Could you check a few things on this drawing? It's one solid part, dimensions in mm from its lowest x, y, z. Coordinates: 2 decimals unless noted, no trailing zeros. Loops run counter-clockwise (first coordinate to the right, second up) from the corner with the lowest first, then second, coordinate; pieces in that order, holes last.
1) Will these pins go through, and if not, where does the flat tip stop? P1, Ø1.2, axis at x = 28.09, z = 19.61, coming from the +Y side; P2, Ø3, axis at x = 29.5, z = 16.5, coming from the +Y side.
2) Imagine slicing it at D-D on x = 29.5. Please give me the cut outline in (y, z).
3) Imagine slicing it at B-B on x = 16.5. Please give me the cut outline in (y, z).
4) Imagine slicing it at A-A on z = 16.5. Please give me the cut outline in (x, y).
5) Imagine slicing it at C-C on z = 3.5. Please give me the cut outline in (x, y).
6) If I drill on line 1 along Z through (x, y) = (29, 0.55) (1 decimal); line 2 along Z through (x, y) = (16, 0.3) (1 decimal); line 3 along X through (y, z) = (0.7, 30.5), over which ranges is the centre line in solid material (lowest first)?
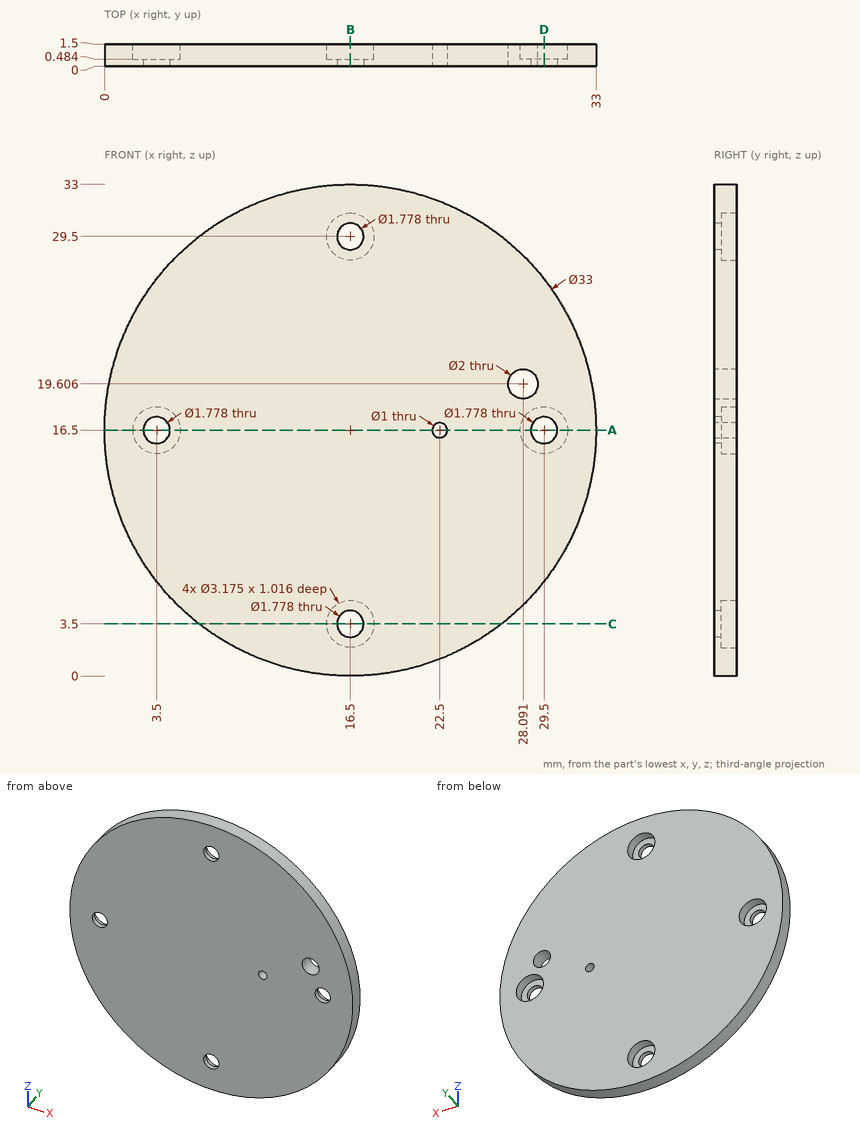
Filled in:
1. P1: passes through
1. P2: stops at y = 0.48
2. outline: (0, 6.34) - (1.5, 6.34) - (1.5, 14.91) - (0.48, 14.91) - (0.48, 15.61) - (0, 15.61) - close; (0, 17.39) - (0.48, 17.39) - (0.48, 18.09) - (1.5, 18.09) - (1.5, 26.66) - (0, 26.66) - close
3. outline: (0, 0) - (1.5, 0) - (1.5, 1.91) - (0.48, 1.91) - (0.48, 2.61) - (0, 2.61) - close; (0, 4.39) - (0.48, 4.39) - (0.48, 5.09) - (1.5, 5.09) - (1.5, 27.91) - (0.48, 27.91) - (0.48, 28.61) - (0, 28.61) - close; (0, 30.39) - (0.48, 30.39) - (0.48, 31.09) - (1.5, 31.09) - (1.5, 33) - (0, 33) - close
4. outline: (0, 0) - (2.61, 0) - (2.61, 0.48) - (1.91, 0.48) - (1.91, 1.5) - (0, 1.5) - close; (4.39, 0) - (22, 0) - (22, 1.5) - (5.09, 1.5) - (5.09, 0.48) - (4.39, 0.48) - close; (23, 0) - (28.61, 0) - (28.61, 0.48) - (27.91, 0.48) - (27.91, 1.5) - (23, 1.5) - close; (30.39, 0) - (33, 0) - (33, 1.5) - (31.09, 1.5) - (31.09, 0.48) - (30.39, 0.48) - close
5. outline: (6.34, 0) - (15.61, 0) - (15.61, 0.48) - (14.91, 0.48) - (14.91, 1.5) - (6.34, 1.5) - close; (17.39, 0) - (26.66, 0) - (26.66, 1.5) - (18.09, 1.5) - (18.09, 0.48) - (17.39, 0.48) - close
6. line 1: z = 5.7 to 15, 18 to 19.2, 20 to 27.3
6. line 2: z = 0 to 2.8, 4.2 to 28.8, 30.2 to 33
6. line 3: x = 7.77 to 15.27, 17.73 to 25.23
